Geometry: final body of the model. Coordinates: model frame, mm. Give positions to 0.01 mm unless a question says otherwise; leave off trailing zeros. Write each loop counter-clockwise with the first axis right and the second up, starting at its lowest first coordinate (ties: lowest second). Pieces come first, ordered by that corner, then holes. Notation, with made-up numbers: M 87.25,3 L 123.25,3 A12 ccw 123.25,7 Z; hole C -26,-10 d7. An arc over 180 degrees is marked long. Use one line per item in the form item = value. Start each with the question number.
Item 1: Section query B-B on y = 361. Return loops of the section in (x, z) (3 decimals), then the cut area to 3 significant figures.
Item 2: Material intervals for line 1 along X through (y, z) = (99.5, 0.2); line 2 along Y through (x, z) = (533.5, 1.55); line 3 along X through (y, z) = (476, 1.05), sorted ascending. Write a range as from..to.
Item 3: Section query C-C on z = 2.55. Give the number of separate pieces and of enclosed holes in the cut face, then the cut area to 3 significant figures.
Item 4: Pull-direction query (Y, two-part tool) for faces 1 (the cylindrical face through (497.61, 289.676, 1.565)), 2 (the flat face through (526, 259, 3.175)); classes: released by +Y, released by -Y, zero draft, split by the parting line, or undercut.
Item 5: Section query A-A on x = 533.4. Return loops of the section in (y, z) (3 decimals), then the cut area to 3 significant figures.
from build123d import *

# Parameters (mm, degrees)
SKETCH1_W                   = 1066.8
SKETCH1_H                   = 654.05
SKETCH1_R                   = 165.1
BOSS_EXTRUDE1_DEPTH         = 3.175
F_1_4_0_25_DIAMETER_HOLE2_D = 6.35
FILLET1_R                   = 3.175


with BuildPart() as part:
    # Sketch1 → Boss-Extrude1 (new body)
    with BuildSketch(Plane.XY):
        with Locations((533.4, 327.025)):
            Rectangle(SKETCH1_W, SKETCH1_H)
        with Locations((533.4, 450.85)):
            Circle(SKETCH1_R, mode=Mode.SUBTRACT)
    extrude(amount=BOSS_EXTRUDE1_DEPTH)

    # 1/4 (0.25) Diameter Hole2 (through all)
    with Locations(Plane(origin=(0, 0, 0), x_dir=(-1, 0, 0), z_dir=(0, 0, -1))):
        with Locations((-998.5375, 555.625), (-998.5375, 98.425), (-68.2625, 98.425), (-68.2625, 555.625)):
            Hole(F_1_4_0_25_DIAMETER_HOLE2_D / 2)

    # Fillet1
    fillet1_edges = [part.edges().sort_by_distance(p)[0] for p in [
        (0, 654.05, 1.5875),
        (1066.8, 654.05, 1.5875),
        (1066.8, 0, 1.5875),
        (0, 0, 1.5875),
    ]]
    fillet(fillet1_edges, radius=FILLET1_R)


solid = part.part
Answer sheet:
q1.outline = M 0,0 L 394.89,0 L 394.89,3.175 L 0,3.175 Z; M 671.91,0 L 1066.8,0 L 1066.8,3.175 L 671.91,3.175 Z
q1.area = 2,510 mm2
q2.line_1 = 0..65.28, 71.25..995.55, 1001.52..1066.8
q2.line_2 = 0..285.75, 615.95..654.05
q2.line_3 = 0..370.23, 696.57..1066.8
q3.separate_pieces = 1
q3.enclosed_holes = 5
q3.area = 612,000 mm2
q4.face_1 = undercut
q4.face_2 = zero draft
q5.outline = M 0,0 L 285.75,0 L 285.75,3.175 L 0,3.175 Z; M 615.95,0 L 654.05,0 L 654.05,3.175 L 615.95,3.175 Z
q5.area = 1,030 mm2
